Part print with two shaded views. Sizes in mm from the minimum x, y, z corner. Coordinates: 2 decimals unless noted, no trailing zeros. Loops run counter-clockwise (first coordinate to the right, second up) from the corner with the lowest first, then second, coordinate; pieces in that order, holes last. Notation, with made-up numbers: (87, -36.75) -> (98, -36.75) arc R25 ccw to (98, -18.75) -> close; hole circle Ø11 at (43.25, -3). An arc over 180 degrees is marked (long way). Return JSON: item names as keys, results as strings. Group by question number.
(1) Saw through at A-A on y = 1.35. Write the cut outline in (x, z).
(2) Saw through at B-B on x = 15.5. Write the cut outline in (y, z).
(3) Probe L1, parallel to Z at x = 15.5, y = 1.9; L2, parallel to Z at x = 15.5, y = 0.85; L3, parallel to X at y = 0.35, z = 3.25. List the from-to ranges inside material, lowest first.
(4) Saw through at C-C on z = 10.5. Write the cut outline in (x, y).
(5) Mould opens along Z. For the marked faces 1, 2, 3 and 4 say: pulls with the +Z half, pulls with the -Z half, needs draft (parallel to the pull), parting line crosses it, or undercut.
(6) Saw through at D-D on y = 0.45. Write the cut outline in (x, z), then the cut area to 3 significant figures.
(7) Flat gauge pins, fed straight in: pin 1 Ø2.5 at (x, z) = (4.5, 4.5) entering from -Y; pin 2 Ø5 at (x, z) = (4.5, 4.5) entering from -Y; pin 3 Ø1 at (x, z) = (7.5, 3.5) entering from -Y; pin 4 Ø4.5 at (x, z) = (15.5, 10.5) entering from -Y. Where does each tip first touch, or does it go through?
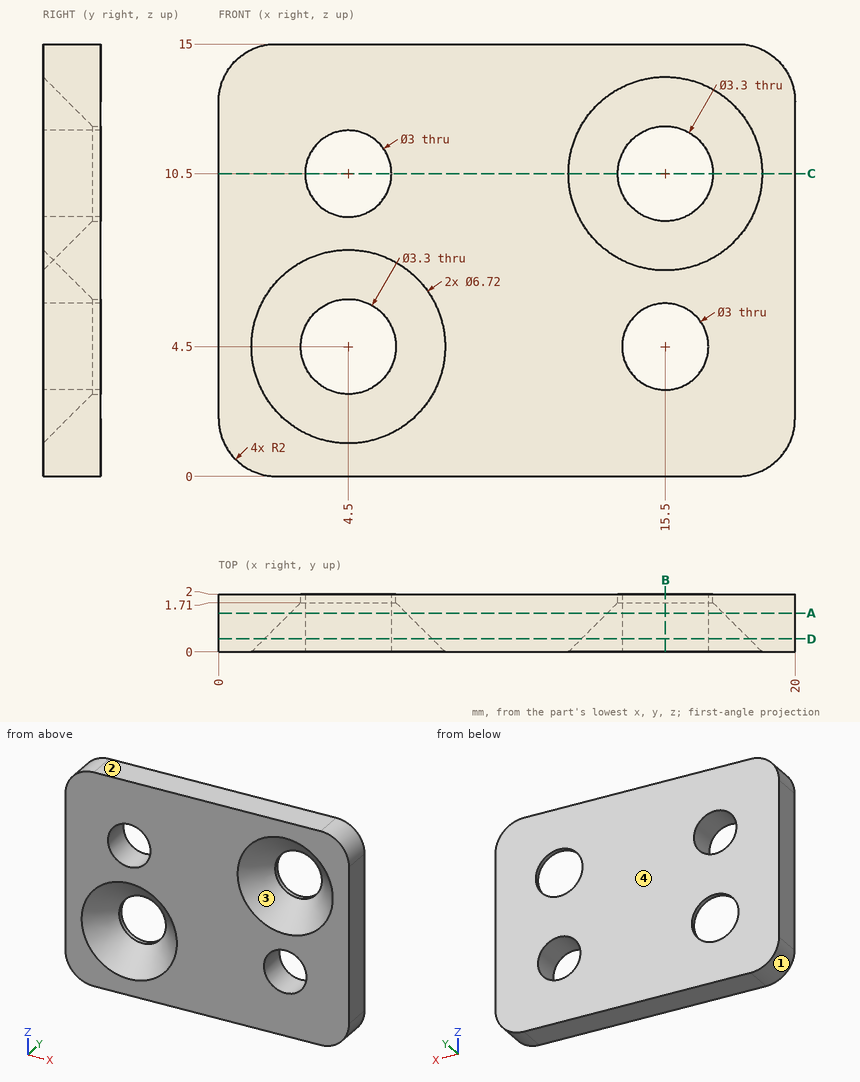
Geometry results:
{
 "1": {"outline": "(0, 2) arc R2 ccw to (2, 0) -> (18, 0) arc R2 ccw to (20, 2) -> (20, 13) arc R2 ccw to (18, 15) -> (2, 15) arc R2 ccw to (0, 13) -> close; hole circle Ø4.02 at (4.5, 4.5); hole circle Ø3 at (4.5, 10.5); hole circle Ø4.02 at (15.5, 10.5); hole circle Ø3 at (15.5, 4.5)"},
 "2": {"outline": "(0, 0) -> (2, 0) -> (2, 3) -> (0, 3) -> close; (0, 6) -> (2, 6) -> (2, 8.85) -> (1.71, 8.85) -> (0, 7.14) -> close; (0, 13.86) -> (1.71, 12.15) -> (2, 12.15) -> (2, 15) -> (0, 15) -> close"},
 "3": {"L1": "0 to 3, 6 to 8.85, 12.15 to 15", "L2": "0 to 3, 6 to 7.99, 13.01 to 15", "L3": "0 to 1.76, 7.24 to 14.67, 16.33 to 20"},
 "4": {"outline": "(0, 0) -> (3, 0) -> (3, 2) -> (0, 2) -> close; (6, 0) -> (12.14, 0) -> (13.85, 1.71) -> (13.85, 2) -> (6, 2) -> close; (17.15, 1.71) -> (18.86, 0) -> (20, 0) -> (20, 2) -> (17.15, 2) -> close"},
 "5": {"face 1": "pulls with the -Z half", "face 2": "pulls with the +Z half", "face 3": "undercut", "face 4": "needs draft"},
 "6": {"outline": "(0, 2) arc R2 ccw to (2, 0) -> (18, 0) arc R2 ccw to (20, 2) -> (20, 13) arc R2 ccw to (18, 15) -> (2, 15) arc R2 ccw to (0, 13) -> close; hole circle Ø5.82 at (4.5, 4.5); hole circle Ø3 at (4.5, 10.5); hole circle Ø5.82 at (15.5, 10.5); hole circle Ø3 at (15.5, 4.5)", "area": "229 mm²"},
 "7": {"pin 1": "through", "pin 2": "y = 0.86", "pin 3": "y = 0", "pin 4": "y = 1.11"}
}
